Autodesk Inventor part; units mm, degrees
ref_plane "YZ Plane" through (0, 0, 0) normal (1, 0, 0) x (0, 1, 0)
ref_plane "XZ Plane" through (0, 0, 0) normal (0, 1, 0) x (-1, 0, 0)
ref_plane "XY Plane" through (0, 0, 0) normal (0, 0, 1) x (1, 0, 0)
sketch "Sketch1" plane through (0, 0, 0) normal (0, 0, 1) x (1, 0, 0)
  circle A0 centre (0, 0) radius 2.0828
  dimension "d0" = 4.1656
extrude "Extrusion1" add sketch "Sketch1" along normal blind 3.175
sketch "Sketch2" plane through (0, 0, 0) normal (0, 1, 0) x (-1, 0, 0)
  line L0 (0, 0) -> (0, -2.2098)
  line L1 (0, 0) -> (3.7016, 0)
  line L2 (0, -2.2098) -> (2.286, -2.2098)
  line L3 (3.7016, 0) -> (3.7016, 3.8864) construction
  arc A0 (3.9368, -0.3736) -> (3.7016, 0) centre (3.7016, -0.2608) ccw
  arc A1 (2.286, -2.2098) -> (3.9368, -0.3736) centre (-0.0192, 1.5228) ccw
  line L4 (3.9624, 0.6553) -> (3.9624, -0.2608) construction
  dimension "d3" = 2.2098
  dimension "d6" = 2.286
  dimension "d12" = 3.9624
revolve "Revolution1" add sketch "Sketch2" angle 360 about axis through (0, 0, 0) along (0, 0, -1)
sketch "Sketch3" plane through (0, 0, -2.2098) normal (0, 0, -1) x (-1, 0, 0)
  circle A0 centre (0, 0) radius 2.286
  line L0 (-0.6874, 1.1906) -> (0.6874, 1.1906)
  line L1 (0.6874, 1.1906) -> (1.3748, 0)
  line L2 (1.3748, 0) -> (0.6874, -1.1906)
  line L3 (0.6874, -1.1906) -> (-0.6874, -1.1906)
  line L4 (-0.6874, -1.1906) -> (-1.3748, 0)
  line L5 (-1.3748, 0) -> (-0.6874, 1.1906)
  dimension "d8" = 2.3813
extrude "Extrusion2" cut sketch "Sketch3" against normal blind 1.5875 contours L0 L1 L2 L3 L4 L5
chamfer "Chamfer1" distance 0.508 angle 45 1 edges at (-2.0828, 0, 3.175)
thread "Thread1"
properties part number "10-32 x438 button head" material "Steel"
Geometry check sheet. Reference: the model listing, model coordinates, mm. A direction names the side the tool comes from. Round coordinates to 2 decimals unless told otherwise and drop trailing zeros. Loops run counter-clockwise (first coordinate to the right, second up) from the corner with the lowest first, then second, coordinate; pieces in that order, holes last. Notation, with made-up numbers: (30.5, 49) -> (59.5, 49) arc R27 cw to (59.5, 84) -> close; hole circle Ø10 at (4, 22). An arc over 180 degrees is marked (long way). Use a Markdown table: item, result.
(1) Set-up check for faces 4 (the flat face through (-1, -1, -2.21)), 5 (the flat face through (-1.03, 0.6, -1.43)), 6 (the flat face through (-2, -2, 0)): record each of +Z, -Z, +X, -X, +Y, -Y from which the full face is reachable in a straight line by a thin tool's end or side.
Calculated:
| item | result |
|---|---|
| face 4 | -Z, +X, -X, +Y, -Y |
| face 5 | -Z |
| face 6 | +Z |
(2) Sectioned sample at A-A (z = 1.6). Enter the section's corners in (x, y).
Calculated:
| item | result |
|---|---|
| outline | circle Ø4.17 at (0, 0) |
(3) Mould release check, pull along X, two halves, no side actions. Record for faces 1 (the flat face through (0, 0, 3.175)), 2 (the flat face through (0, 1.191, -1)), 3 (the cylindrical face through (1.987, -0.626, 1.315)): released by +X, released by -X, zero draft, split by the parting line, or undercut.
Calculated:
| item | result |
|---|---|
| face 1 | zero draft |
| face 2 | undercut |
| face 3 | split by the parting line |
(4) Sectioned sample at B-B (z = 2.8). Enter the section's corners in (x, y), then the cut area to 3 significant figures.
Calculated:
| item | result |
|---|---|
| outline | circle Ø3.9 at (0, 0) |
| area | 11.9 mm² |
(5) Scan lines: probe 1 along Y at (x, z) = (1, -1.15); probe 2 along X at (y, z) = (1, -1.55); probe 3 along Y at (x, z) = (-0.5, -0.7). Record each from-to range of solid material in increasing order.
Calculated:
| item | result |
|---|---|
| probe 1 | -3.31 to -0.65, 0.65 to 3.31 |
| probe 2 | -2.95 to -0.8, 0.8 to 2.95 |
| probe 3 | -3.73 to -1.19, 1.19 to 3.73 |
(6) Go/stop test with flat-tipped pins: P1, Ø0.7, axis at x = 0.5, z = -1, coming from the -Y side; P2, Ø1.1, axis at x = 0, z = -1, coming from the +Y side; P3, Ø2.5, axis at x = 0, y = 0.5, coming from the -Z side; P4, Ø1.5, axis at x = -1.5, z = 0, coming from the -Y side. Record where each tip stops, or that it passes through.
Calculated:
| item | result |
|---|---|
| P1 | y = -3.76 |
| P2 | y = 3.9 |
| P3 | z = -2.21 |
| P4 | y = -3.88 |
